Autodesk Fusion 360 part; units mm, degrees
sketch "Sketch1" plane through (0, 0, 0) normal (0, 1, 0) x (1, 0, 0)
  line L0 (-42.5, 0) -> (42.5, 0)
  line L1 (-42.5, 3) -> (42.5, 3)
  line L2 (42.5, -3) -> (-42.5, -3)
  circle A0 centre (-42.5, 0) radius 1.65
  circle A1 centre (-42.5, 0) radius 3
  circle A2 centre (42.5, 0) radius 3
  circle A3 centre (42.5, 0) radius 1.65
  dimension "d1" = 85
  dimension "d8" = 3.3
  dimension "d9" = 6
  dimension "d10" = 3.3
extrude "Extrude1" add sketch "Sketch1" along normal blind 3
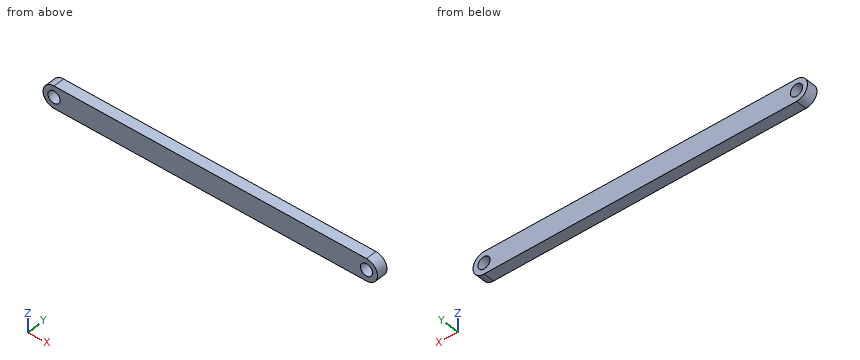
Input: part model. Units: mm. Frame: model coordinates. Coordinates: 2 decimals unless noted, no trailing zeros. Loops run counter-clockwise (first coordinate to the right, second up) from the corner with the lowest first, then second, coordinate; pieces in that order, holes last. Notation, with made-up numbers: (69.25, 13.25) -> (90.25, 13.25) arc R14 cw to (90.25, 34.25) -> close; hole circle Ø10 at (28.25, 71.25). An arc over 180 degrees is marked (long way). Write each question's results on one line, items separated by ' | '. Start each with the question number.
Q1. Ray query, line 1 (X direction, y = 0.6, z = 0); line 2 (Z direction, x = -42.5, y = 1.5); line 3 (X direction, y = 2.45, z = 0.6). Return the intervals inside material, ascending. Write a range as from..to.
Q2. Pin query (flat end, axial travel): pin 1 (1.5 mm diameter, centred on y = 1, z = -2.5, fed in from +X); pin 2 (1.5 mm diameter, centred on y = 1.5, z = 2, fed in from +X). Return the tip coordinate at first contact, or that it passes through.
Q3. Section B-B, the plane y = 1.3. Return the cut outline in (x, z).
Q4. Section A-A, the plane z = 0. Return the cut outline in (x, y), plus the area to 3 significant figures.
Found:
1) line 1: -45.5..-44.15, -40.85..40.85, 44.15..45.5 | line 2: -3..-1.65, 1.65..3 | line 3: -45.44..-44.04, -40.96..40.96, 44.04..45.44
2) pin 1: x = 44.94 | pin 2: x = 45.23
3) outline: (-42.5, -3) -> (42.5, -3) arc R3 ccw to (42.5, 3) -> (-42.5, 3) arc R3 ccw to start; hole circle Ø3.3 at (-42.5, 0); hole circle Ø3.3 at (42.5, 0)
4) outline: (-45.5, 0) -> (-44.15, 0) -> (-44.15, 3) -> (-45.5, 3) -> close; (-40.85, 0) -> (40.85, 0) -> (40.85, 3) -> (-40.85, 3) -> close; (44.15, 0) -> (45.5, 0) -> (45.5, 3) -> (44.15, 3) -> close | area: 253 mm2
